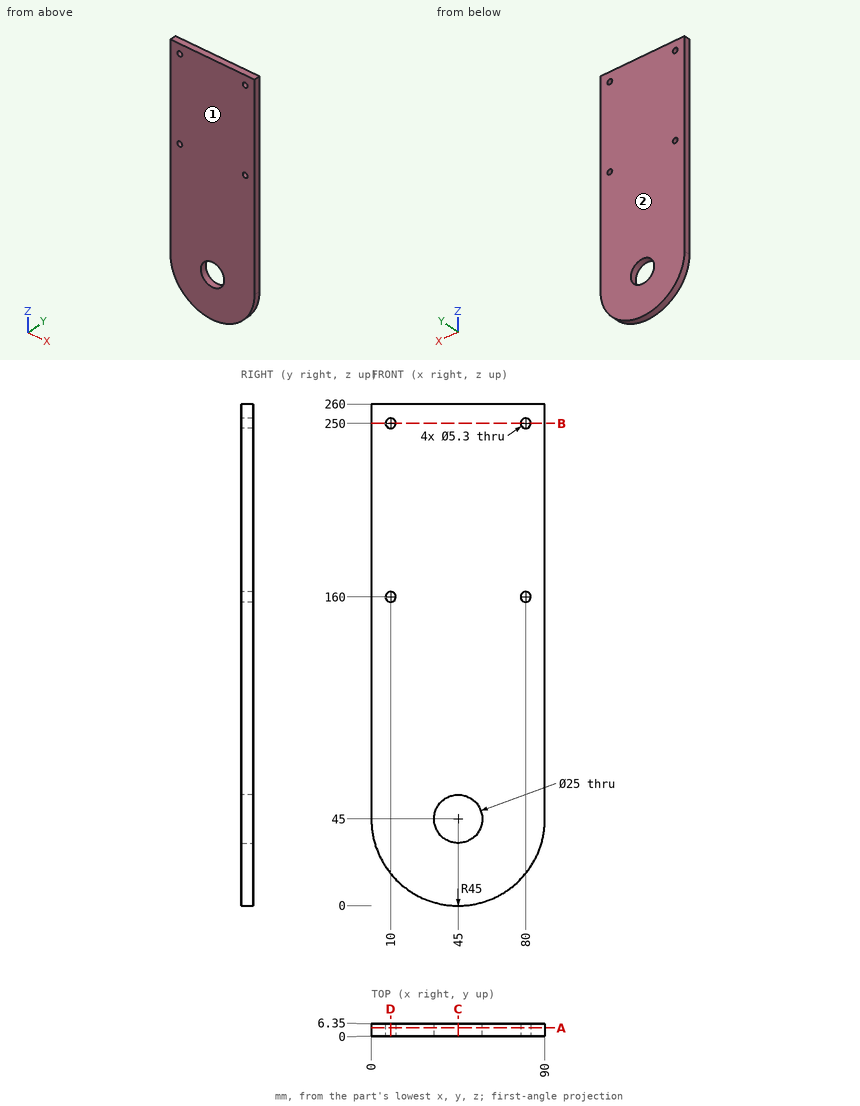
Drawing for the job (mm, zero at the part's lowest x, y, z). Coordinates: 2 decimals unless noted, no trailing zeros. Order: outer loops, then holes, each group sorted by start corner. A loop starts at its lowest first (then second) coordinate and runs counter-clockwise, first axis right, second up. Notation, with made-up numbers: (15, 68) -> (74, 68) arc R34 ccw to (74, 101) -> close; hole circle Ø4 at (20, -27). An arc over 180 degrees is marked (long way). One line per item, written item: value.
(1) Slice it at D-D, the plane x = 10. List the corners of the cut face in (y, z), plus the area to 3 significant figures.
Checked values:
outline: (0, 16.72) -> (6.35, 16.72) -> (6.35, 157.35) -> (0, 157.35) -> close; (0, 162.65) -> (6.35, 162.65) -> (6.35, 247.35) -> (0, 247.35) -> close; (0, 252.65) -> (6.35, 252.65) -> (6.35, 260) -> (0, 260) -> close
area: 1,480 mm2
(2) Slice it at B-B, the plane z = 250. List the corners of the cut face in (x, y).
Checked values:
outline: (0, 0) -> (7.35, 0) -> (7.35, 6.35) -> (0, 6.35) -> close; (12.65, 0) -> (77.35, 0) -> (77.35, 6.35) -> (12.65, 6.35) -> close; (82.65, 0) -> (90, 0) -> (90, 6.35) -> (82.65, 6.35) -> close
(3) Drop flat-ended pins along their axis: pin 1 Ø7 at (x, z) = (10, 250) entering from -Y; pin 2 Ø1.5 at (x, y) = (46, 3) entering from -Z. Give the stop position or say it passes through.
Checked values:
pin 1: y = 0
pin 2: z = 0
(4) Probe line 1 (X direction, y = 1.75, z = 250); line 2 (X direction, y = 4.75, z = 42); line 3 (X direction, y = 6.25, z = 43.5) (3 decimals). List the from-to ranges inside material, lowest first. Write a range as [from, to].
Checked values:
line 1: [0, 7.35], [12.65, 77.35], [82.65, 90]
line 2: [0.1, 32.87], [57.13, 89.9]
line 3: [0.025, 32.59], [57.41, 89.975]
(5) Slice it at A-A, the plane y = 4.25. List the corners of the cut face in (x, z).
Checked values:
outline: (0, 45) arc R45 ccw to (90, 45) -> (90, 260) -> (0, 260) -> close; hole circle Ø5.3 at (10, 160); hole circle Ø5.3 at (10, 250); hole circle Ø25 at (45, 45); hole circle Ø5.3 at (80, 160); hole circle Ø5.3 at (80, 250)
(6) Slice it at C-C, the plane x = 45. List the corners of the cut face in (y, z), plus the area to 3 significant figures.
Checked values:
outline: (0, 0) -> (6.35, 0) -> (6.35, 32.5) -> (0, 32.5) -> close; (0, 57.5) -> (6.35, 57.5) -> (6.35, 260) -> (0, 260) -> close
area: 1,490 mm2
(7) Mould opens along Y. For the marked faces 1 and 2 say: pulls with the +Y half, pulls with the -Y half, needs draft (parallel to the pull), parting line crosses it, or undercut.
Checked values:
face 1: pulls with the -Y half
face 2: pulls with the +Y half
